from build123d import *

# Parameters (mm, degrees)
TAPA_CAJA_PLACAS_SALIENTE_DEPTH = 7.5


with BuildPart() as part:
    # Tapa-Caja-Placas-Croquis → Tapa-Caja-Placas-Saliente (new body)
    with BuildSketch(Plane(origin=(0, 0, 0), x_dir=(1, 0, 0), z_dir=(0, 1, 0))):
        Polygon((-26, -1.25), (-23.5, -1.25), (-23.5, -2.5), (-24.75, -2.5), (-24.75, -3.75), (-23.5, -3.75), (23.5, -3.75), (24.75, -3.75), (24.75, -2.5), (23.5, -2.5), (23.5, -1.25), (26, -1.25), (27.25, -1.25), (27.25, 0), (26, 0), (26, 1.25), (-26, 1.25), (-26, 0), (-27.25, 0), (-27.25, -1.25), align=None)
    extrude(amount=TAPA_CAJA_PLACAS_SALIENTE_DEPTH)


solid = part.part
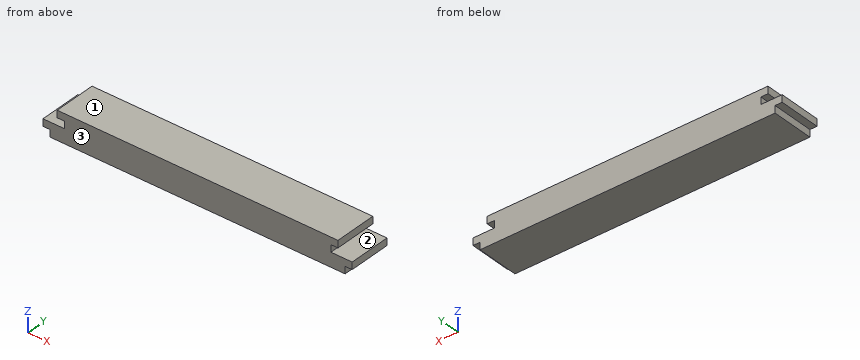
Check sheet for the modelled part. Datum: model origin and axes. Units: mm. Face numbers are marked on the shaded views. Round coordinates to 2 decimals unless told otherwise and drop trailing zeros. Loops run counter-clockwise (first coordinate to the right, second up) from the corner with the lowest first, then second, coordinate; pieces in that order, holes last. Notation, with made-up numbers: (-7.75, 9) -> (22.25, 9) arc R5 ccw to (22.25, 16) -> close; hole circle Ø1 at (64.25, -5.5). An arc over 180 degrees is marked (long way). Put each result on its own line as item: value. Start each with the question number.
1. Section check A-A (y = 5.5). Enter the section's corners in (x, z).
2. Draft check along Z on the marked faces 1, 2 and 3. Enter one of: +Z half, -Z half, draft (parallel to the pull), parting line (faces both ways), or undercut.
3. Section check B-B (z = 3.15). Enter the section's corners in (x, y).
4. Scan lines: probe 1 along Z at (x, y) = (24, 2.25); probe 2 along X at (y, z) = (5, -0.05); probe 3 along X at (y, z) = (1, 1.85). Record each from-to range of solid material in increasing order.
5. Gauge pin test, flat ends, axial feed: pin 1 (0.6 mm diameter, centred on y = 4.5, z = 3.5, fed in from +X); pin 2 (0.6 mm diameter, centred on y = 5.5, z = 2, fed in from -X); pin 3 (1.1 mm diameter, centred on x = 26, y = 3.5, fed in from +Z). Record the tip position at first contact, or that the pin passes through.
Findings:
1. outline: (-27.25, 0) -> (-26, 0) -> (-26, -1.25) -> (26, -1.25) -> (26, 0) -> (27.25, 0) -> (27.25, 1.25) -> (23.5, 1.25) -> (23.5, 2.5) -> (24.75, 2.5) -> (24.75, 3.75) -> (-24.75, 3.75) -> (-24.75, 2.5) -> (-23.5, 2.5) -> (-23.5, 1.25) -> (-27.25, 1.25) -> close
2. face 1: +Z half
2. face 2: undercut
2. face 3: draft
3. outline: (-24.75, 0) -> (24.75, 0) -> (24.75, 7.5) -> (-24.75, 7.5) -> close
4. probe 1: z = -1.25 to 1.25, 2.5 to 3.75
4. probe 2: x = -26 to 26
4. probe 3: x = -23.5 to 23.5
5. pin 1: stops at x = 24.75
5. pin 2: stops at x = -23.5
5. pin 3: stops at z = 1.25
